Input: part model. Units: mm. Frame: model coordinates. Give positions to 0.01 mm unless a question says otherwise; leave off trailing zeros. Loops run counter-clockwise (first coordinate to the right, second up) from the corner with the lowest first, then second, coordinate; pieces in that order, holes last. Notation, with made-up numbers: (36, -29.5) -> (56, -29.5) arc R12 cw to (56, -25.5) -> close; hole circle Ø10 at (63, -3). An arc over 180 degrees is marked (long way). Answer as a JSON object with one key per item and string values. Group by question number.
```python
from build123d import *


with BuildPart() as part:
    # Sketch1 → Revolução1 (revolve)
    with BuildSketch(Plane.XY, mode=Mode.PRIVATE) as revolu_o1_sk:
        with BuildLine():
            Line((0, 26.9), (0, 22.65))
            Line((0, 22.65), (3.913688674, 22.65))
            ThreePointArc((3.913688674, 22.65), (8, 24.6595), (12.086311326, 22.65))
            Line((12.086311326, 22.65), (16, 22.65))
            Line((16, 22.65), (16, 26.9))
            ThreePointArc((16, 26.9), (15.677817459, 27.677817459), (14.9, 28))
            Line((14.9, 28), (1.1, 28))
            ThreePointArc((1.1, 28), (0.322182541, 27.677817459), (0, 26.9))
        make_face()
    revolve(revolu_o1_sk.sketch.rotate(Axis((200, 0, 0), (-1, 0, 0)), 270), axis=Axis((200, 0, 0), (-1, 0, 0)))


solid = part.part
```
Q1. Pin query (flat end, axial travel): pin 1 Ø3 at (x, y) = (10, 9.5) entering from -Z; pin 2 Ø6 at (x, y) = (13.5, 17.5) entering from +Z; pin 3 Ø3 at (x, y) = (2.5, -17) entering from +Z. Return the tip coordinate at first contact, or that it passes through.
Q2. Section C-C on x = 5. Return the cut outline in (y, z).
Q3. Ray query, probe 1 along Y at (x, z) = (13, 0); probe 2 along Y at (x, z) = (12.5, -16.5); probe 3 along Z at (x, y) = (10.5, 11). Return the intervals inside material, ascending.
Q4. Pull-direction query (Z, two-part tool) for faces 1 (the face through (7.903, -27.334, -6.07)), 2 (the face through (16, -18, 14)), 3 (the face through (1.984, -13.782, -17.974)); classes: +Z half, -Z half, draft (parallel to the pull), parting line (faces both ways), or undercut.
Q5. Section A-A on y = 0. Return the cut outline in (x, z).
Numbers:
{
 "1": {"pin 1": "stops at z = -26.83", "pin 2": "stops at z = 23.95", "pin 3": "stops at z = 23.32"},
 "2": {"outline": "circle Ø56 at (0, 0); hole circle Ø47.4 at (0, 0)"},
 "3": {"probe 1": "y = -28 to -22.65, 22.65 to 28", "probe 2": "y = -22.62 to -15.52, 15.52 to 22.62", "probe 3": "z = -25.75 to -21.35, 21.35 to 25.75"},
 "4": {"face 1": "parting line", "face 2": "draft", "face 3": "undercut"},
 "5": {"outline": "(0, -26.9) arc R1.1 ccw to (1.1, -28) -> (14.9, -28) arc R1.1 ccw to (16, -26.9) -> (16, -22.65) -> (12.09, -22.65) arc R5.16 cw to (3.91, -22.65) -> (0, -22.65) -> close; (0, 22.65) -> (3.91, 22.65) arc R5.16 cw to (12.09, 22.65) -> (16, 22.65) -> (16, 26.9) arc R1.1 ccw to (14.9, 28) -> (1.1, 28) arc R1.1 ccw to (0, 26.9) -> close"}
}
